Autodesk Inventor part; units mm, degrees
ref_plane "YZ Plane" through (0, 0, 0) normal (1, 0, 0) x (0, 1, 0)
ref_plane "XZ Plane" through (0, 0, 0) normal (0, 1, 0) x (-1, 0, 0)
ref_plane "XY Plane" through (0, 0, 0) normal (0, 0, 1) x (1, 0, 0)
sketch "Sketch2" plane through (0, 0, 0) normal (0, 1, 0) x (-1, 0, 0)
  line L0 (44.45, 63.5) -> (-44.45, 63.5)
  line L1 (-44.45, 63.5) -> (-44.45, -63.5)
  line L2 (-44.45, -63.5) -> (44.45, -63.5)
  line L3 (44.45, -63.5) -> (44.45, 63.5)
  line L4 (44.45, 63.5) -> (-44.45, -63.5) construction
  line L5 (-44.45, 63.5) -> (44.45, -63.5) construction
  point P0 (0, 0)
  dimension "d0" = 127
  dimension "d1" = 88.9
extrude "Extrusion1" add sketch "Sketch2" against normal blind 4.7625
sketch "Sketch4" plane through (0, 0, 0) normal (0, 1, 0) x (1, 0, 0)
  line L0 (-44.45, -63.5) -> (-44.45, 63.5)
  line L1 (44.45, 63.5) -> (44.45, -63.5)
  line L2 (-44.45, 63.5) -> (44.45, 63.5)
  line L3 (44.45, 63.5) -> (44.45, 58.7375)
  line L4 (44.45, 58.7375) -> (-44.45, 58.7375)
  line L5 (-44.45, 58.7375) -> (-44.45, 63.5)
  point P0 (0, 0)
  point P1 (-44.45, 58.7375)
  dimension "d4" = 4.7625
extrude "Extrusion2" add sketch "Sketch4" along normal blind 38.1
sketch "Sketch5" plane through (0, 0, 0) normal (0, 1, 0) x (1, 0, 0)
  line L0 (44.45, -63.5) -> (-44.45, -63.5)
  line L1 (-44.45, 58.7375) -> (44.45, 58.7375)
  line L2 (-44.45, -63.5) -> (-41.275, -63.5)
  line L3 (-41.275, -63.5) -> (-41.275, 58.7375)
  line L4 (-44.45, 58.7375) -> (-44.45, -63.5)
  line L5 (44.45, 63.5) -> (44.45, -63.5)
  line L6 (44.45, -63.5) -> (41.275, -63.5)
  line L7 (-44.45, 58.7375) -> (-44.45, -63.5)
  line L8 (-44.45, -63.5) -> (-44.45, 63.5)
  line L9 (-44.45, 58.7375) -> (-44.45, 63.5)
  line L10 (-44.45, 63.5) -> (-41.275, 63.5)
  line L11 (-44.45, 63.5) -> (44.45, 63.5)
  line L12 (-41.275, 58.7375) -> (-41.275, 63.5)
  line L13 (44.45, 58.7375) -> (-44.45, 58.7375)
  point P0 (0, 0)
  point P1 (-44.45, 58.7375)
  point P2 (41.275, 63.5)
  dimension "d7" = 3.175
extrude "Extrusion3" add sketch "Sketch5" along normal blind 38.1
sketch "Sketch6" plane through (0, 0, 0) normal (0, 1, 0) x (1, 0, 0)
  line L0 (-41.275, -63.5) -> (41.275, -63.5)
  line L1 (-41.275, 58.7375) -> (41.275, 58.7375)
  line L2 (-22.225, -63.5) -> (-19.05, -63.5)
  line L3 (-19.05, -63.5) -> (-19.05, 58.7375)
  line L4 (-19.05, 58.7375) -> (-22.225, 58.7375)
  line L5 (-22.225, 58.7375) -> (-22.225, -63.5)
  line L6 (0, -63.5) -> (3.175, -63.5)
  line L7 (3.175, -63.5) -> (3.175, 58.7375)
  line L8 (3.175, 58.7375) -> (0, 58.7375)
  line L9 (0, 58.7375) -> (0, -63.5)
  line L10 (15.875, -63.5) -> (19.05, -63.5)
  line L11 (19.05, -63.5) -> (19.05, 58.7375)
  line L12 (19.05, 58.7375) -> (15.875, 58.7375)
  line L13 (15.875, 58.7375) -> (15.875, -63.5)
  line L14 (-41.275, -63.5) -> (-41.275, 58.7375)
  point P0 (0, 0)
  point P1 (15.875, -63.5)
  point P2 (19.05, -63.5)
  point P3 (19.05, 58.7375)
  point P4 (0, 58.7375)
  point P5 (0, -63.5)
  point P6 (3.175, -63.5)
  dimension "d11" = 3.175
  dimension "d12" = 3.175
  dimension "d13" = 3.175
  dimension "d49" = 19.05
  dimension "d50" = 19.05
  dimension "d51" = 12.7
extrude "Extrusion4" add sketch "Sketch6" along normal blind 38.1 contours L5 L1 L3 L0 | L9 L1 L7 L0 | L13 L1 L11 L0
sketch "Sketch9" plane through (44.45, -4.7625, 63.5) normal (1, 0, 0) x (0, 0, -1)
  line L0 (0, 0) -> (0, 42.8625)
  line L1 (127, 0) -> (127, 42.8625)
  line L2 (0, 0) -> (127, 0)
  line L3 (127, 0) -> (127, 4.7625)
  line L4 (127, 4.7625) -> (0, 4.7625)
  line L5 (0, 4.7625) -> (0, 0)
  point P0 (63.5, 4.7625)
  dimension "d37" = 4.7625
extrude "Extrusion5" add sketch "Sketch9" along normal blind 101.6
sketch "Sketch10" plane through (44.45, 38.1, 63.5) normal (1, 0, 0) x (0, 0, -1)
  line L0 (127, -38.1) -> (127, 0)
  line L1 (122.2375, 0) -> (0, 0)
  line L2 (127, -38.1) -> (122.2375, -38.1)
  line L3 (122.2375, -38.1) -> (122.2375, 0)
  line L4 (122.2375, 0) -> (127, 0)
  line L5 (127, 0) -> (127, -38.1)
  point P0 (63.5, -38.1)
extrude "Extrusion6" add sketch "Sketch10" along normal blind 101.6
equation "\"d0\" = depth"
equation "\"d1\" = width"
equation "\"d2\" = baseThickness"
equation "\"d4\" = backThickness"
equation "\"d5\" = backHeight"
equation "\"d7\" = edgeThickness"
equation "\"d9\" = edgeHeight"
equation "\"d11\" = dividerThickness"
equation "\"d12\" = dividerThickness"
equation "\"d13\" = dividerThickness"
equation "\"d19\" = dividerHeight"
equation "\"d37\" = baseThickness"
equation "\"d38\" = waterShelfWidth"
equation "\"d40\" = waterShelfWidth"
equation "\"baseThickness\" = 4.7625"
equation "\"width\" = 88.9"
equation "\"depth\" = 127"
equation "\"backHeight\" = 38.1"
equation "\"backThickness\" = 4.7625"
equation "\"edgeThickness\" = 3.175"
equation "\"edgeHeight\" = 38.1"
equation "\"dividerThickness\" = 3.175"
equation "\"dividerHeight\" = 38.1"
equation "\"waterShelfWidth\" = 101.6"
properties part number "shelfForElectronicsV01"
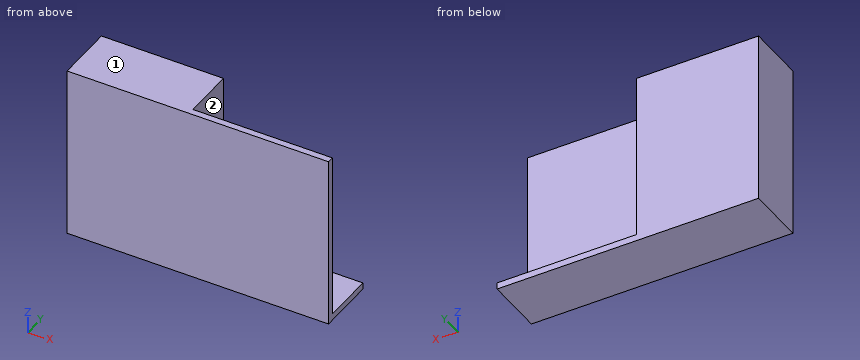
Design review of the part built by this model. Coordinates are the model's own, in mm. Face numbers are marked on the shaded views. A direction names the side the tool comes from. Round coordinates to 2 decimals unless told otherwise and drop trailing zeros. Loops run counter-clockwise (first coordinate to the right, second up) from the corner with the lowest first, then second, coordinate; pieces in that order, holes last. Notation, with made-up numbers: M -27.75,3 L 17.25,3 A13 ccw 17.25,23 Z; hole C 29.25,-22.5 d9. An arc over 180 degrees is marked long. Answer as a JSON object with one key per item and string values.
Item 1: Machinability: for the marked faces 1 and 2, which of the approach directions +Z, -Z, +X, -X, +Y, -Y give a long, thin tool a straight path to every point of the face, cutting with its end or side? Answer none if there is none.
Answer sheet:
{"face 1": "+Z, +X, -X, +Y, -Y", "face 2": "+Z, +X, +Y"}
Item 2: We need section B-B on z = 17. Give the boundary of the cut face in (x, y).
Answer sheet:
{"outline": "M -44.45,-4.76 L 146.05,-4.76 L 146.05,0 L 44.45,0 L 44.45,38.1 L -44.45,38.1 Z"}
Item 3: Clearance check with flat-ended pins moving along their axes: P1, Ø11.5, axis at x = 111.5, y = 18, coming from the +Z side; P2, Ø1.5, axis at y = 26.5, z = 27, coming from the +X side. State where each tip first meets the part, or that it passes through.
Answer sheet:
{"P1": "stops at z = -58.74", "P2": "stops at x = 44.45"}
Item 4: We need section A-A on y = 3. Give the boundary of the cut face in (x, z).
Answer sheet:
{"outline": "M -44.45,-63.5 L 146.05,-63.5 L 146.05,-58.74 L 44.45,-58.74 L 44.45,63.5 L -44.45,63.5 Z"}
Item 5: Wall thickness on L1, parallel to Y at x = 73, z = -49; L2, parallel to Z at x = 48, y = 26; L3, parallel to X at y = 25, z = -19: over which ranges is each line inside the solid? List them lowest first. Write a range as from..to.
Answer sheet:
{"L1": "y = -4.76..0", "L2": "z = -63.5..-58.74", "L3": "x = -44.45..44.45"}
